Source: CAD feature listing. Evaluate the final solid. Frame: model axes, mm. Face numbers are marked on the shaded views. Coordinates: 2 decimals unless noted, no trailing zeros. Order: outer loops, then holes, each group sorted by start corner. A loop starts at its lowest first (then second) coordinate and runs counter-clockwise, first axis right, second up. Notation, with made-up numbers: (7.25, 56) -> (21.25, 56) arc R24 ccw to (21.25, 72) -> close; hole circle Ø2 at (34.25, -23). An arc over 180 degrees is marked (long way). Write item = value, one per line. Start each with the question number.
Item 1: Section query A-A (y = 0). Output: boundary loops of the cut face in (x, z), then the cut area to 3 significant figures.
Item 2: Mould query, pull axis X, two halves, no side actions, for the marked faces 1 and 2. Classes: released by +X, released by -X, zero draft, split by the parting line, or undercut.
Item 3: Section query D-D (y = -11.5). Output: boundary loops of the cut face in (x, z).
Item 4: Ray query, line 1 along X through (y, z) = (0, -15.5); line 2 along Y through (x, z) = (0, 13); line 3 along X through (y, z) = (4, 19.5). Return the intervals inside material, ascending. Write a range as [from, to].
Item 5: Contact query for flat-ended pins moving along their axis: pin 1 (4 mm diameter, centred on y = -7.5, z = 9.5, fed in from -X); pin 2 (5 mm diameter, centred on x = 11.5, z = 15, fed in from -Y); pin 3 (6 mm diameter, centred on x = 1.5, y = -7, fed in from -Z); pin 4 (5 mm diameter, centred on x = -8.5, z = -17, fed in from -Y). Output: stop coordinate, or through.
Item 6: Section query B-B (x = 0). Output: boundary loops of the cut face in (y, z).
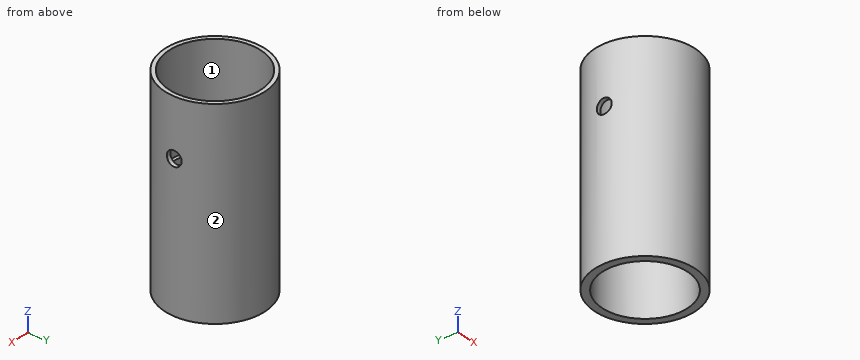
```python
from build123d import *

# Parameters (mm, degrees)
F0_R     = 15
F0_R_2   = 13.5
F1_DEPTH = 30
F0_R_3   = 12.5
F2_DEPTH = 30
F3_R     = 2.2347042808
F4_DEPTH = 50
F5_R     = 13.75
F6_DEPTH = 30
F7_R     = 12.75
F8_DEPTH = 30


with BuildPart() as f1:
    # F0 (on Top) → F1 (new body)
    with BuildSketch(Plane.XY):
        Circle(F0_R)
        Circle(F0_R_2, mode=Mode.SUBTRACT)
    extrude(amount=F1_DEPTH)

    # F0 (on Top) → F2 (join)
    with BuildSketch(Plane.XY):
        Circle(F0_R)
        Circle(F0_R_2, mode=Mode.SUBTRACT)
        Circle(F0_R_2)
        Circle(F0_R_3, mode=Mode.SUBTRACT)
    extrude(amount=-F2_DEPTH)

    # F3 (on Right) → F4 (cut, symmetric)
    with BuildSketch(Plane.YZ):
        with Locations((0, 13)):
            Circle(F3_R)
    extrude(amount=F4_DEPTH, both=True, mode=Mode.SUBTRACT)

    # F5 (on face) → F6 (cut)
    with BuildSketch(Plane.XY.offset(30)):
        Circle(F5_R)
    extrude(amount=-F6_DEPTH, mode=Mode.SUBTRACT)

    # F7 (on face) → F8 (cut)
    with BuildSketch(Plane(origin=(0, 0, -30), x_dir=(1, 0, 0), z_dir=(0, 0, -1))):
        Circle(F7_R)
    extrude(amount=-F8_DEPTH, mode=Mode.SUBTRACT)


solid = f1.part
```
Computed:
q1.outline = (-15, -30) -> (-12.75, -30) -> (-12.75, 0) -> (-13.75, 0) -> (-13.75, 10.77) -> (-15, 10.77) -> close; (-15, 15.23) -> (-13.75, 15.23) -> (-13.75, 30) -> (-15, 30) -> close; (12.75, -30) -> (15, -30) -> (15, 10.77) -> (13.75, 10.77) -> (13.75, 0) -> (12.75, 0) -> close; (13.75, 15.23) -> (15, 15.23) -> (15, 30) -> (13.75, 30) -> close
q1.area = 199 mm^2
q2.face_1 = undercut
q2.face_2 = split by the parting line
q3.outline = (-9.63, -30) -> (-5.51, -30) -> (-5.51, 0) -> (-7.54, 0) -> (-7.54, 30) -> (-9.63, 30) -> close; (5.51, -30) -> (9.63, -30) -> (9.63, 30) -> (7.54, 30) -> (7.54, 0) -> (5.51, 0) -> close
q4.line_1 = [-15, -12.75], [12.75, 15]
q4.line_2 = [-15, -13.75], [13.75, 15]
q4.line_3 = [-14.46, -13.16], [13.16, 14.46]
q5.pin_1 = -13.96
q5.pin_2 = -12
q5.pin_3 = through
q5.pin_4 = -13.75
q6.outline = (-15, -30) -> (-12.75, -30) -> (-12.75, 0) -> (-13.75, 0) -> (-13.75, 30) -> (-15, 30) -> close; (12.75, -30) -> (15, -30) -> (15, 30) -> (13.75, 30) -> (13.75, 0) -> (12.75, 0) -> close
